The listing builds one solid part. Answer for the finished solid, in the listing's coordinates (mm). A direction names the side the tool comes from. Round coordinates to 2 decimals unless told otherwise and drop trailing zeros.
(1) For faces 1 (the face through (-127, -6, -69.176)), 2 (the face through (126, -6, -69.176)), 3 (the face through (39, -6, 6.61)), determine the directions among +Z, -Z, +X, -X, +Y, -Y from which every point of the face is accessible in a straight line to the end or side of a thin tool.
(2) The mould has two halves that part along X. Classify faces 4 (the face through (-242.59, -3.62, 79.55)), 5 (the face through (-39, -6, 6.61)): +X half, -X half, draft (parallel to the pull), parting line (faces both ways), or undercut.
(3) Each of these flat-tipped pins is pushed along its axis until it touches: pin 1 Ø1.5 at (x, y) = (55.5, -7) entering from -Z; pin 2 Ø2 at (y, z) = (-2, 60.5) entering from +X; pin 3 Ø1.5 at (y, z) = (-9, -58.5) entering from +X. Where does it stop, or does it pass through?
(4) Find the intervals of material crossed by probe 1 along X at (y, z) = (-3, 23); probe 2 along X at (y, z) = (-5.5, 43); probe 3 along X at (y, z) = (-0.75, -25), in increasing order.
from build123d import *

# Parameters (mm, degrees)
F1_DEPTH = 12.7
F2_R     = 12.69999
F3_R     = 12.69999


# Not quite as in the source:
# - a fillet or chamfer is up to 0.001 mm smaller than in the source, because OpenCascade refuses the exact size


with BuildPart() as f1:
    # F0 (on Front) → F1 (new body)
    with BuildSketch(Plane.XZ):
        with BuildLine():
            add(Edge.make_bspline(
                [(0, 22.1556201577), (4.6081906185, 22.4393960088), (8.8232094422, 21.4276518673), (12.0959098929, 19.0737502837)],
                knots=[0, 0, 0, 0, 12.4823458556, 12.4823458556, 12.4823458556, 12.4823458556], degree=3))
            add(Edge.make_bspline(
                [(0, 22.1556201577), (-4.6081906185, 22.4393960088), (-8.8232094422, 21.4276518673), (-12.0959098929, 19.0737502837)],
                knots=[0, 0, 0, 0, 12.4823458556, 12.4823458556, 12.4823458556, 12.4823458556], degree=3))
            Line((-12.0959098929, 19.0737502837), (-17.7139695734, 43.9015217125))
            Line((-17.7139695734, 43.9015217125), (-25.8638337255, 6.609717384))
            Line((-25.8638337255, 6.609717384), (-52.1656684577, 6.609717384))
            add(Edge.make_bspline(
                [(-52.1656684577, 6.609717384), (-60.3978514517, 6.5219254793), (-78.5756597545, 6.3269402408), (-116.4466347426, 8.1732890136), (-162.2561628931, 52.1737802861), (-162.6985337077, 74.2627820904), (-162.8867536783, 83.3681735719)],
                knots=[0, 0, 0, 0, 0.2084568336, 0.4601327492, 0.7768832352, 1, 1, 1, 1], degree=3))
            Line((-162.8867536783, 83.3681735719), (-320.8426764241, 83.3681735719))
            add(Edge.make_bspline(
                [(-320.8426764241, 83.3681735719), (-310.9533159528, 77.5358259805), (-288.6959219459, 64.6452840474), (-244.3194495003, 36.5716752771), (-184.7380258313, -6.777248073), (-199.2239955574, -48.5914785577), (-206.0440058214, -69.0696899563)],
                knots=[0, 0, 0, 0, 0.2057375573, 0.4598387655, 0.7366005134, 1, 1, 1, 1], degree=3))
            Line((-206.0440058214, -69.0696899563), (-152.1980017424, -69.1764205694))
            Line((-152.1980017424, -69.1764205694), (-100.3352329135, -69.1764205694))
            add(Edge.make_bspline(
                [(-100.3352329135, -69.1764205694), (-93.1837151487, -69.1338341935), (-75.4005733711, -70.292076661), (-27.8541687884, -63.5387172898), (-12.4442655786, -120.211944878), (0, -135.5760842562)],
                knots=[0, 0, 0, 0, 0.2530200956, 0.5731929838, 1, 1, 1, 1], degree=3))
            add(Edge.make_bspline(
                [(100.3352329135, -69.1764205694), (93.1837151487, -69.1338341935), (75.4005733711, -70.292076661), (27.8541687884, -63.5387172898), (12.4442655786, -120.211944878), (0, -135.5760842562)],
                knots=[0, 0, 0, 0, 0.2530200956, 0.5731929838, 1, 1, 1, 1], degree=3))
            Line((100.3352329135, -69.1764205694), (152.1980017424, -69.1764205694))
            Line((152.1980017424, -69.1764205694), (206.0440058214, -69.0696899563))
            add(Edge.make_bspline(
                [(320.8426764241, 83.3681735719), (310.9533159528, 77.5358259805), (288.6959219459, 64.6452840474), (244.3194495003, 36.5716752771), (184.7380258313, -6.777248073), (199.2239955574, -48.5914785577), (206.0440058214, -69.0696899563)],
                knots=[0, 0, 0, 0, 0.2057375573, 0.4598387655, 0.7366005134, 1, 1, 1, 1], degree=3))
            Line((320.8426764241, 83.3681735719), (162.8867536783, 83.3681735719))
            add(Edge.make_bspline(
                [(52.1656684577, 6.609717384), (60.3978514517, 6.5219254793), (78.5756597545, 6.3269402408), (116.4466347426, 8.1732890136), (162.2561628931, 52.1737802861), (162.6985337077, 74.2627820904), (162.8867536783, 83.3681735719)],
                knots=[0, 0, 0, 0, 0.2084568336, 0.4601327492, 0.7768832352, 1, 1, 1, 1], degree=3))
            Line((52.1656684577, 6.609717384), (25.8638337255, 6.609717384))
            Line((25.8638337255, 6.609717384), (17.7139695734, 43.9015217125))
            Line((17.7139695734, 43.9015217125), (12.0959098929, 19.0737502837))
        make_face()
    extrude(amount=F1_DEPTH)

    # F2 (radius 12.7 in the source; OpenCascade refuses exactly that, so slightly less here)
    f2_edges = [f1.edges().sort_by_distance(p)[0] for p in [
        (241.864715, 0, 83.368174),
    ]]
    fillet(f2_edges, radius=F2_R)

    # F3 (radius 12.7 in the source; OpenCascade refuses exactly that, so slightly less here)
    f3_edges = [f1.edges().sort_by_distance(p)[0] for p in [
        (-241.864715, 0, 83.368174),
    ]]
    fillet(f3_edges, radius=F3_R)


solid = f1.part
Solutions:
1. face 1: -Z, -X, +Y, -Y
1. face 2: -Z, +X, +Y, -Y
1. face 3: +Z, +Y, -Y
2. face 4: draft
2. face 5: undercut
3. pin 1: stops at z = -68.82
3. pin 2: stops at x = 284.09
3. pin 3: stops at x = 202.8
4. probe 1: x = -226.59 to -128.72, -22.28 to -12.98, 12.98 to 22.28, 128.72 to 226.59
4. probe 2: x = -255.13 to -149.34, -17.91 to -17.51, 17.51 to 17.91, 149.34 to 255.13
4. probe 3: x = -195.9 to 195.9
